For this review, take the finished solid that the model builds, in its own axes (mm). A direction names the side the tool comes from. Give positions to 0.01 mm unless a question says otherwise; leave off trailing zeros. Write each loop counter-clockwise with the first axis right and the second up, starting at its lowest first coordinate (ties: lowest second). Pieces come first, ordered by that corner, then holes. Notation, with made-up numbers: (-17.75, 2.5) -> (39.25, 2.5) arc R14 cw to (39.25, 13.5) -> close; hole circle Ø7 at (72.25, -9.5). An arc over 180 degrees is marked (long way). Return JSON: item names as keys, results as strings.
from build123d import *

# Parameters (mm, degrees)
F0_W          = 4.19
F0_H          = 40.08
F2_DEPTH      = 2.54
F1_W          = 3.5
F1_H          = 8
F3_DEPTH      = 5.08
F4_R          = 1.524
F5_R          = 1.524
F6_R          = 1.524
F7_W          = 7.7873766422
F7_H          = 11.2617432605
F8_DEPTH      = 5
F8_DEPTH_BACK = 5


with BuildPart() as f2:
    # F0 (on Top) → F2 (new body)
    with BuildSketch(Plane.XY):
        Rectangle(F0_W, F0_H)
    extrude(amount=F2_DEPTH)

    # F1 (on Top) → F3 (join)
    with BuildSketch(Plane.XY):
        with Locations((0, 7.8411972237)):
            Rectangle(F1_W, F1_H)
        with Locations((0, -7.3970568238)):
            Rectangle(F1_W, F1_H)
    extrude(amount=F3_DEPTH)

    # F4
    f4_edges = [f2.edges().sort_by_distance(p)[0] for p in [
        (-1.75, 11.841197, 3.81),
    ]]
    fillet(f4_edges, radius=F4_R)

    # F5
    f5_edges = [f2.edges().sort_by_distance(p)[0] for p in [
        (1.75, 11.841197, 3.81),
        (1.75, 3.841197, 3.81),
        (1.75, -3.397057, 3.81),
        (1.75, -11.397057, 3.81),
        (-1.75, 3.841197, 3.81),
        (-1.75, -11.397057, 3.81),
        (-1.75, -3.397057, 3.81),
    ]]
    fillet(f5_edges, radius=F5_R)

    # F6
    f6_edges = [f2.edges().sort_by_distance(p)[0] for p in [
        (-2.095, 20.04, 1.27),
        (2.095, 20.04, 1.27),
        (2.095, -20.04, 1.27),
        (-2.095, -20.04, 1.27),
    ]]
    fillet(f6_edges, radius=F6_R)

    # F7 (on Right) → F8 (join, two sides)
    with BuildSketch(Plane.YZ) as f8_sk:
        with Locations((-23.6965231597, 1.3423765777)):
            Rectangle(F7_W, F7_H)
    extrude(amount=-F8_DEPTH)
    extrude(f8_sk.sketch, amount=F8_DEPTH_BACK)


solid = f2.part
1. For pin 1 (3 mm diameter, centred on y = 3.5, z = 2, fed in from +X) (3 decimals); pin 2 (1.8 mm diameter, centred on x = 0.5, y = -6.5, fed in from +Z); pin 3 (0.8 mm diameter, centred on y = -8.5, z = 3.5, fed in from -X); pin 4 (1.5 mm diameter, centred on y = -12, z = -1, fed in from -X) (1 decimal), all flat-tipped, find the tip position at first contact; note any pin that passes through.
Results found:
{"pin 1": "stops at x = 2.095", "pin 2": "stops at z = 5.08", "pin 3": "stops at x = -1.75", "pin 4": "passes through"}
2. The part is to be moulded in two halves that separate along Y. For faces 1 (the cylindrical face through (1.292, -10.962, 3.828)), 2 (the cylindrical face through (-1.66, 19.58, 1.29)), 3 (the flat face through (-2.095, 0, 1)), 4 (the cylindrical face through (1.32, -3.86, 3.83)), say which applies: +Y half, -Y half, draft (parallel to the pull), parting line (faces both ways), or undercut.
Results found:
{"face 1": "undercut", "face 2": "+Y half", "face 3": "draft", "face 4": "undercut"}
3. To check wall thickness, follow probe 1 along Y at (x, z) = (-2.75, 4.5); probe 2 along Z at (x, y) = (-1.25, -9.5); probe 3 along Z at (x, y) = (1.25, -2). State the ranges of each line that lie inside material, in increasing order.
Results found:
{"probe 1": "y = -27.59 to -19.8", "probe 2": "z = 0 to 5.08", "probe 3": "z = 0 to 2.54"}
4. Add section C-C, the plane z = 0.75. State the section outline as (x, y) points (3 decimals).
Results found:
{"outline": "(-5, -27.59) -> (5, -27.59) -> (5, -19.803) -> (1.387, -19.803) arc R1.524 ccw to (2.095, -18.516) -> (2.095, 18.516) arc R1.524 ccw to (0.571, 20.04) -> (-0.571, 20.04) arc R1.524 ccw to (-2.095, 18.516) -> (-2.095, -18.516) arc R1.524 ccw to (-1.387, -19.803) -> (-5, -19.803) -> close"}
5. Add section B-B, the plane y = -8. State the section outline as (x, z) points (3 decimals), plus the area to 3 significant figures.
Results found:
{"outline": "(-2.095, 0) -> (2.095, 0) -> (2.095, 2.54) -> (1.75, 2.54) -> (1.75, 5.08) -> (-1.75, 5.08) -> (-1.75, 2.54) -> (-2.095, 2.54) -> close", "area": "19.5 mm²"}
6. Add section A-A, the plane z = 3.5. State the section outline as (x, y) points, plus the area to 3 significant figures.
Results found:
{"outline": "(-5, -27.59) -> (5, -27.59) -> (5, -19.8) -> (-5, -19.8) -> close; (-1.75, -9.87) arc R1.52 ccw to (-0.23, -11.4) -> (0.23, -11.4) arc R1.52 ccw to (1.75, -9.87) -> (1.75, -4.92) arc R1.52 ccw to (0.23, -3.4) -> (-0.23, -3.4) arc R1.52 ccw to (-1.75, -4.92) -> close; (-1.75, 5.37) arc R1.52 ccw to (-0.23, 3.84) -> (0.23, 3.84) arc R1.52 ccw to (1.75, 5.37) -> (1.75, 10.32) arc R1.52 ccw to (0.23, 11.84) -> (-0.23, 11.84) arc R1.52 ccw to (-1.75, 10.32) -> close", "area": "130 mm²"}
7. Add section D-D, the plane x = 2.75. State the section outline as (y, z) points, plus the area to 3 significant figures.
Results found:
{"outline": "(-27.59, -4.29) -> (-19.8, -4.29) -> (-19.8, 6.97) -> (-27.59, 6.97) -> close", "area": "87.7 mm²"}
8. For faces 5 (the flat face through (0, 0, 0)), 6 (the flat face through (-1.75, 8, 4)), 7 (the cylindrical face through (-1.315, 4.299, 3.828)), 8 (the flat face through (0, 8, 5.08)), 9 (the cylindrical face through (1.3, 11.4, 3.8)), list the 3-axis set-ups (+Z, -Z, +X, -X, +Y, -Y) from which the entire face can be reached by the end or side of a thin tool; tool diameter is ignored.
Results found:
{"face 5": "-Z, +X, -X, +Y", "face 6": "+Z, -X, +Y", "face 7": "+Z, -X", "face 8": "+Z, +X, -X, +Y", "face 9": "+Z, +X, +Y"}
